Autodesk Inventor part; units mm, degrees
ref_plane "Work Plane1" through (0, 14, -10) normal (0, 0, 1) x (1, 0, 0)
ref_plane "YZ Plane" through (0, 0, 0) normal (1, 0, 0) x (0, 1, 0)
ref_plane "XZ Plane" through (0, 0, 0) normal (0, 1, 0) x (-1, 0, 0)
sketch "Sketch1" plane through (0, 0, 0) normal (0, 1, 0) x (-1, 0, 0)
  line L0 (0, 25) -> (0, 13) construction
  line L1 (3, 25) -> (3, 13)
  line L2 (-3, 13) -> (-3, 25)
  arc A0 (3, 25) -> (-3, 25) centre (0, 25) ccw
  arc A1 (-3, 13) -> (3, 13) centre (0, 13) ccw
  line L3 (0, 30.2784) -> (0, -34.8413) construction
  line L4 (24.1166, 0) -> (-17.2731, 0) construction
  line L5 (0, 10) -> (0, -10)
  line L6 (3, -25) -> (3, -13)
  line L7 (-3, -13) -> (-3, -25)
  arc A2 (-3, -25) -> (3, -25) centre (0, -25) ccw
  arc A3 (3, -13) -> (-3, -13) centre (0, -13) ccw
  point P0 (0, 0)
  point P1 (0, 19)
  dimension "d0" = 12
  dimension "d1" = 3
  dimension "d2" = 20
extrude "Extrusion1" add sketch "Sketch1" along normal blind 14 contours A3 L6 A2 L7
ref_plane "Work Plane1" through (0, 14, -10) normal (0, 0, 1) x (1, 0, 0)
sketch "Sketch2" plane through (0, 14, -10) normal (0, 0, 1) x (1, 0, 0)
  circle A0 centre (0, -7) radius 1.5
  line L0 (3, 0) -> (-3, 0)
  line L1 (3, -14) -> (-3, -14)
  line L2 (3, -14) -> (3, 0)
  line L3 (-3, -14) -> (-3, 0)
  point P0 (0, -14)
  dimension "d5" = 3
  dimension "d6" = 7
  dimension "d7" = 3
extrude "Extrusion2" add sketch "Sketch2" along normal blind 25 and the other way blind 2 contours A0
sketch "Sketch3" plane through (0, 7, 15) normal (0, 0, 1) x (1, 0, 0)
  circle A0 centre (0, 0) radius 1.5
  circle A1 centre (0, 0) radius 1.5
  circle A2 centre (0, 0) radius 1.25
  point P0 (0, -7)
  dimension "d12" = 2.5
extrude "Extrusion3" cut sketch "Sketch3" against normal blind 5
properties part number "paletas"
Input: part model. Units: mm. Frame: model coordinates. A direction names the side the tool comes from. Coordinates: 2 decimals unless noted, no trailing zeros. Loops run counter-clockwise (first coordinate to the right, second up) from the corner with the lowest first, then second, coordinate; pieces in that order, holes last. Notation, with made-up numbers: M -35,-14.75 L -8,-14.75 A30 ccw -8,12.25 Z; hole C 27.5,-17.5 d3. An arc over 180 degrees is marked long. Use a Markdown table: item, result. Add a question column.
1) Draft query along X for faces 1 (the flat face through (3, 7, -19)), 2 (the flat face through (0, 0, -19)), 3 (the cylindrical face through (0, 7, -28)). Return one class per face: +X half, -X half, draft (parallel to the pull), parting line (faces both ways), or undercut.
2) Section C-C, the plane z = 10.5. Return the cut outline in (x, y), plus the area to 3 significant figures.
3) Set-up query: faces 4 (the flat face through (-3, 7, -19)), 5 (the cylindrical face through (-0.27, 5.78, 12.54)). Return all of +Z, -Z, +X, -X, +Y, -Y with unobstructed straight access to the full face (end or side cutting, diameter ignored); none if empty.
4) Line query: L1, parallel to Z at x = -2.5, y = 6; L2, parallel to Z at x = 0.5, y = 12.25; L3, parallel to Y at x = 0.25, z = -8. Output: solid intervals per line, ascending. Write a range as from..to.
5) Pin query (flat end, axial travel): P1, Ø1.5, axis at x = 1, z = 0.5, coming from the +Y side; P2, Ø1.5, axis at y = 3.5, z = 3.5, coming from the +X side; P3, Ø3, axis at x = -1.5, y = 11, coming from the +Z side; P4, Ø1.5, axis at y = 5.5, z = -2, coming from the -X side. Return the tip coordinate at first contact, or that it passes through.
6) Section D-D, the plane y = 9.5. Return the cut outline in (x, z), plus the area to 3 significant figures.
7) Section A-A, the plane y = 7. Return the cut outline in (x, z).
8) Section B-B, the plane x = 0. Return the cut outline in (y, z).
Answer below:
| question | item | result |
|---|---|---|
| 1 | face 1 | +X half |
| 1 | face 2 | draft |
| 1 | face 3 | parting line |
| 2 | outline | C 0,7 d2.5 |
| 2 | area | 4.91 mm2 |
| 3 | face 4 | +Z, -Z, -X, +Y, -Y |
| 3 | face 5 | +Z |
| 4 | L1 | -26.66..-11.34 |
| 4 | L2 | -27.96..-10.04 |
| 4 | L3 | 5.52..8.48 |
| 5 | P1 | y = 8.48 |
| 5 | P2 | through |
| 5 | P3 | z = -10 |
| 5 | P4 | x = -1.3 |
| 6 | outline | M -3,-25 A3 ccw 3,-25 L 3,-13 A3 ccw -3,-13 Z |
| 6 | area | 100 mm2 |
| 7 | outline | M -3,-25 A3 ccw 3,-25 L 3,-13 A3 ccw 1.5,-10.4 L 1.5,10 L 1.25,10 L 1.25,15 L -1.25,15 L -1.25,10 L -1.5,10 L -1.5,-10.4 A3 ccw -3,-13 Z |
| 8 | outline | M 0,-28 L 14,-28 L 14,-10 L 8.5,-10 L 8.5,10 L 8.25,10 L 8.25,15 L 5.75,15 L 5.75,10 L 5.5,10 L 5.5,-10 L 0,-10 Z |
